Autodesk Inventor part; units mm, degrees
ref_plane "Work Plane1" through (0, 0, 5) normal (0, 0, 1) x (1, 0, 0)
ref_plane "YZ Plane" through (0, 0, 0) normal (1, 0, 0) x (0, 1, 0)
ref_plane "XZ Plane" through (0, 0, 0) normal (0, 1, 0) x (-1, 0, 0)
sketch "Sketch1" plane through (0, 0, 0) normal (0, 0, 1) x (1, 0, 0)
  line L0 (14.6962, 12.74) -> (14.6962, 0) construction
  line L1 (10.61, 12.2) -> (1.53, 12.2)
  arc A0 (1.53, 12.2) -> (0, 10.67) centre (1.53, 10.67) ccw
  line L2 (0, 10.67) -> (0, 1.53)
  arc A1 (0, 1.53) -> (1.53, 0) centre (1.53, 1.53) ccw
  line L3 (1.53, 0) -> (10.61, 0)
  arc A2 (10.61, 0) -> (12.14, 1.53) centre (10.61, 1.53) ccw
  arc A3 (12.14, 10.67) -> (10.61, 12.2) centre (10.61, 10.67) ccw
  line L4 (12.14, 10.67) -> (12.14, 1.53)
  point P0 (0, 0)
  point P1 (0, 0)
  dimension "d10" = 12.74
ref_plane "Work Plane1" through (0, 0, 5) normal (0, 0, 1) x (1, 0, 0)
sketch "Sketch2" plane through (0, 0, 5) normal (0, 0, 1) x (1, 0, 0)
  line L0 (10.88, 12.74) -> (1.8, 12.74)
  line L1 (10.88, 12.74) -> (1.8, 12.74)
  arc A0 (1.8, 12.74) -> (0, 10.94) centre (1.8, 10.94) ccw
  line L2 (0, 10.94) -> (0, 1.8)
  arc A1 (0, 1.8) -> (1.8, 0) centre (1.8, 1.8) ccw
  line L3 (1.8, 0) -> (10.88, 0)
  arc A2 (10.88, 0) -> (12.68, 1.8) centre (10.88, 1.8) ccw
  line L4 (12.68, 1.8) -> (12.68, 10.94)
  arc A3 (12.68, 10.94) -> (10.88, 12.74) centre (10.88, 10.94) ccw
  circle A4 centre (6.34, 6.37) radius 2.8
  line L5 (5.665, 8.395) -> (7.015, 8.395)
  line L6 (7.015, 4.345) -> (5.665, 4.345)
  line L7 (5.665, 4.345) -> (7.015, 8.395) construction
  line L8 (5.665, 8.395) -> (7.015, 4.345) construction
  line L9 (8.365, 5.695) -> (8.365, 7.045)
  line L10 (4.315, 7.045) -> (4.315, 5.695)
  line L11 (4.315, 5.695) -> (8.365, 7.045) construction
  line L12 (8.365, 5.695) -> (4.315, 7.045) construction
  line L13 (4.315, 5.695) -> (5.665, 5.695)
  line L14 (7.015, 5.695) -> (8.365, 5.695)
  line L15 (5.665, 4.345) -> (5.665, 5.695)
  line L16 (5.665, 7.045) -> (5.665, 8.395)
  line L17 (8.365, 7.045) -> (7.015, 7.045)
  line L18 (5.665, 7.045) -> (4.315, 7.045)
  line L19 (7.015, 8.395) -> (7.015, 7.045)
  line L20 (7.015, 5.695) -> (7.015, 4.345)
  point P0 (0, 0)
  dimension "d3" = 5.6
  dimension "d4" = 4.05
  dimension "d5" = 1.35
  dimension "d6" = 4.05
  dimension "d7" = 1.35
extrude "Extrusion3" add sketch "Sketch1" along normal blind 5
sketch "Sketch3" plane through (0, 0, 5) normal (0, 0, 1) x (1, 0, 0)
  line L0 (10.61, 12.47) -> (1.53, 12.47)
  line L1 (10.61, 12.47) -> (1.53, 12.47)
  arc A0 (1.53, 12.47) -> (-0.27, 10.67) centre (1.53, 10.67) ccw
  line L2 (-0.27, 10.67) -> (-0.27, 1.53)
  arc A1 (-0.27, 1.53) -> (1.53, -0.27) centre (1.53, 1.53) ccw
  line L3 (1.53, -0.27) -> (10.61, -0.27)
  arc A2 (10.61, -0.27) -> (12.41, 1.53) centre (10.61, 1.53) ccw
  line L4 (12.41, 1.53) -> (12.41, 10.67)
  arc A3 (12.41, 10.67) -> (10.61, 12.47) centre (10.61, 10.67) ccw
  circle A4 centre (6.07, 6.1) radius 2.8
  line L5 (5.395, 8.125) -> (6.745, 8.125)
  line L6 (6.745, 4.075) -> (5.395, 4.075)
  line L7 (5.395, 4.075) -> (6.745, 8.125) construction
  line L8 (5.395, 8.125) -> (6.745, 4.075) construction
  line L9 (8.095, 5.425) -> (8.095, 6.775)
  line L10 (4.045, 6.775) -> (4.045, 5.425)
  line L11 (4.045, 5.425) -> (8.095, 6.775) construction
  line L12 (8.095, 5.425) -> (4.045, 6.775) construction
  line L13 (4.045, 5.425) -> (5.395, 5.425)
  line L14 (6.745, 5.425) -> (8.095, 5.425)
  line L15 (5.395, 4.075) -> (5.395, 5.425)
  line L16 (5.395, 6.775) -> (5.395, 8.125)
  line L17 (8.095, 6.775) -> (6.745, 6.775)
  line L18 (5.395, 6.775) -> (4.045, 6.775)
  line L19 (6.745, 8.125) -> (6.745, 6.775)
  line L20 (6.745, 5.425) -> (6.745, 4.075)
  line L21 (10.61, 12.2) -> (1.53, 12.2)
  line L22 (0, 10.67) -> (0, 1.53)
  point P0 (0, 0)
  point P1 (-0.27, -0.27)
  point P2 (6.07, 12.2)
  point P3 (0, 6.1)
  point P4 (6.07, 6.1)
  dimension "d14" = 5.6
  dimension "d15" = 4.05
  dimension "d16" = 1.35
  dimension "d17" = 4.05
  dimension "d18" = 1.35
extrude "Extrusion4" add sketch "Sketch3" along normal blind 4.8 contours A4
sketch "Sketch4" plane through (0, 0, 0) normal (0, 0, -1) x (-1, 0, 0)
  line L0 (-13.9436, 0) -> (-13.9436, 2.266)
  line L1 (-15.5559, 0) -> (-15.5559, 6.84)
  line L2 (-1.53, 0) -> (-10.61, 0)
  line L3 (-11.5311, 9.89) -> (-0.6089, 9.89) construction
  line L4 (-0.6089, 9.89) -> (-0.6089, 6.84) construction
  line L5 (-0.6089, 6.84) -> (-11.5311, 6.84) construction
  line L6 (-11.5311, 6.84) -> (-11.5311, 9.89) construction
  line L7 (-7.4059, 5.4371) -> (-4.7341, 5.4371) construction
  line L8 (-4.7341, 5.4371) -> (-4.7341, 2.266) construction
  line L9 (-4.7341, 2.266) -> (-7.4059, 2.266) construction
  line L10 (-7.4059, 2.266) -> (-7.4059, 5.4371) construction
  line L11 (-10.6289, 6.84) -> (-10.6289, 9.3092)
  line L12 (-10.6289, 9.3092) -> (-11.5311, 9.3092)
  line L13 (-11.5311, 9.3092) -> (-11.5311, 9.89)
  line L14 (-11.5311, 9.89) -> (-8.9606, 9.89)
  line L15 (-8.9606, 9.89) -> (-8.9606, 9.3092)
  line L16 (-8.9606, 9.3092) -> (-9.8627, 9.3092)
  line L17 (-9.8627, 9.3092) -> (-9.8627, 6.84)
  line L18 (-9.8627, 6.84) -> (-10.6289, 6.84)
  line L19 (-7.1291, 6.84) -> (-8.7703, 6.84)
  line L20 (-8.7703, 6.84) -> (-8.7703, 7.3714)
  line L21 (-8.7703, 7.3714) -> (-8.3328, 7.3714)
  line L22 (-8.3328, 7.3714) -> (-8.3328, 9.3586)
  line L23 (-8.3328, 9.3586) -> (-8.7703, 9.3586)
  line L24 (-8.7703, 9.3586) -> (-8.7703, 9.89)
  line L25 (-8.7703, 9.89) -> (-7.1291, 9.89)
  line L26 (-7.1291, 9.89) -> (-7.1291, 9.3586)
  line L27 (-7.1291, 9.3586) -> (-7.5666, 9.3586)
  line L28 (-7.5666, 9.3586) -> (-7.5666, 7.3714)
  line L29 (-7.5666, 7.3714) -> (-7.1291, 7.3714)
  line L30 (-7.1291, 7.3714) -> (-7.1291, 6.84)
  line L31 (-3.5057, 6.84) -> (-4.2669, 6.84)
  line L32 (-4.2669, 6.84) -> (-4.2669, 8.8618)
  line L33 (-4.2669, 8.8618) -> (-4.8206, 7.5568)
  line L34 (-4.8206, 7.5568) -> (-5.3446, 7.5568)
  line L35 (-5.3446, 7.5568) -> (-5.8982, 8.8618)
  line L36 (-5.8982, 8.8618) -> (-5.8982, 6.84)
  line L37 (-5.8982, 6.84) -> (-6.6199, 6.84)
  line L38 (-6.6199, 6.84) -> (-6.6199, 9.89)
  line L39 (-6.6199, 9.89) -> (-5.7376, 9.89)
  line L40 (-5.7376, 9.89) -> (-5.0603, 8.3848)
  line L41 (-5.0603, 8.3848) -> (-4.3881, 9.89)
  line L42 (-4.3881, 9.89) -> (-3.5057, 9.89)
  line L43 (-3.5057, 9.89) -> (-3.5057, 6.84)
  line L44 (-2.8729, 6.84) -> (-2.8729, 9.89)
  line L45 (-2.8729, 9.89) -> (-0.8116, 9.89)
  line L46 (-0.8116, 9.89) -> (-0.8116, 9.3092)
  line L47 (-0.8116, 9.3092) -> (-2.1117, 9.3092)
  line L48 (-2.1117, 9.3092) -> (-2.1117, 8.7728)
  line L49 (-2.1117, 8.7728) -> (-0.9129, 8.7728)
  line L50 (-0.9129, 8.7728) -> (-0.9129, 8.192)
  line L51 (-0.9129, 8.192) -> (-2.1117, 8.192)
  line L52 (-2.1117, 8.192) -> (-2.1117, 7.4208)
  line L53 (-2.1117, 7.4208) -> (-0.8116, 7.4208)
  line L54 (-0.8116, 7.4208) -> (-0.8116, 6.84)
  line L55 (-0.8116, 6.84) -> (-2.8729, 6.84)
  spline S0 degree 2 poles (-4.8725, 3.3684) (-4.8725, 2.8864) (-5.483, 2.266) (-6.0169, 2.266) knots 0 0 0 1 2 2 2
  spline S1 degree 2 poles (-6.0169, 2.266) (-6.2838, 2.266) (-6.7015, 2.4192) (-6.8473, 2.57) knots 0 0 0 1 2 2 2
  spline S2 degree 2 poles (-6.8473, 2.57) (-7.0203, 2.7455) (-7.2057, 3.3016) (-7.2057, 3.6897) knots 0 0 0 1 2 2 2
  spline S3 degree 2 poles (-7.2057, 3.6897) (-7.2057, 4.0901) (-7.0327, 4.7129) (-6.8374, 4.9527) knots 0 0 0 1 2 2 2
  spline S4 degree 2 poles (-6.8374, 4.9527) (-6.6521, 5.1801) (-6.049, 5.4371) (-5.6362, 5.4371) knots 0 0 0 1 2 2 2
  spline S5 degree 2 poles (-5.6362, 5.4371) (-5.4855, 5.4371) (-5.1839, 5.3976) (-5.1295, 5.3852) knots 0 0 0 1 2 2 2
  line L56 (-5.1295, 5.3852) -> (-5.1295, 4.7871)
  line L57 (-5.1295, 4.7871) -> (-5.1839, 4.7871)
  spline S6 degree 2 poles (-5.1839, 4.7871) (-5.2383, 4.8143) (-5.4855, 4.881) (-5.6436, 4.881) knots 0 0 0 1 2 2 2
  spline S7 degree 2 poles (-5.6436, 4.881) (-6.002, 4.881) (-6.3925, 4.5028) (-6.4395, 4.1519) knots 0 0 0 1 2 2 2
  spline S8 degree 2 poles (-6.4395, 4.1519) (-6.2887, 4.2483) (-5.9798, 4.3619) (-5.7845, 4.3619) knots 0 0 0 1 2 2 2
  spline S9 degree 2 poles (-5.7845, 4.3619) (-5.6189, 4.3619) (-5.3297, 4.273) (-5.2185, 4.1889) knots 0 0 0 1 2 2 2
  spline S10 degree 2 poles (-5.2185, 4.1889) (-5.0603, 4.0678) (-4.8725, 3.6748) (-4.8725, 3.3684) knots 0 0 0 1 2 2 2
  spline S11 degree 2 poles (-5.7648, 2.9086) (-5.7054, 2.9828) (-5.6412, 3.1558) (-5.6412, 3.3313) knots 0 0 0 1 2 2 2
  spline S12 degree 2 poles (-5.6412, 3.3313) (-5.6412, 3.4796) (-5.7153, 3.6724) (-5.7821, 3.7292) knots 0 0 0 1 2 2 2
  spline S13 degree 2 poles (-5.7821, 3.7292) (-5.8513, 3.7885) (-6.0218, 3.8305) (-6.1182, 3.8305) knots 0 0 0 1 2 2 2
  spline S14 degree 2 poles (-6.1182, 3.8305) (-6.1998, 3.8305) (-6.3678, 3.7885) (-6.442, 3.7589) knots 0 0 0 1 2 2 2
  spline S15 degree 2 poles (-6.442, 3.7589) (-6.442, 3.7391) (-6.4469, 3.6452) (-6.4469, 3.5735) knots 0 0 0 1 2 2 2
  spline S16 degree 2 poles (-6.4469, 3.5735) (-6.4469, 3.309) (-6.3555, 2.9902) (-6.2838, 2.9086) knots 0 0 0 1 2 2 2
  spline S17 degree 2 poles (-6.2838, 2.9086) (-6.2319, 2.8419) (-6.0935, 2.785) (-6.0193, 2.785) knots 0 0 0 1 2 2 2
  spline S18 degree 2 poles (-6.0193, 2.785) (-5.9575, 2.785) (-5.8142, 2.8468) (-5.7648, 2.9086) knots 0 0 0 1 2 2 2
  point P0 (0, 0)
  point P1 (-6.07, 0)
  point P2 (-6.07, 2.266)
  point P3 (-6.07, 6.84)
  point P4 (-6.07, 6.84)
  point P5 (-6.07, 2.266)
  dimension "d21" = 2.266
  dimension "d22" = 6.84
extrude "Extrusion5" add sketch "Sketch4" along normal blind 0.9
properties part number "IPC TIME 6 key"
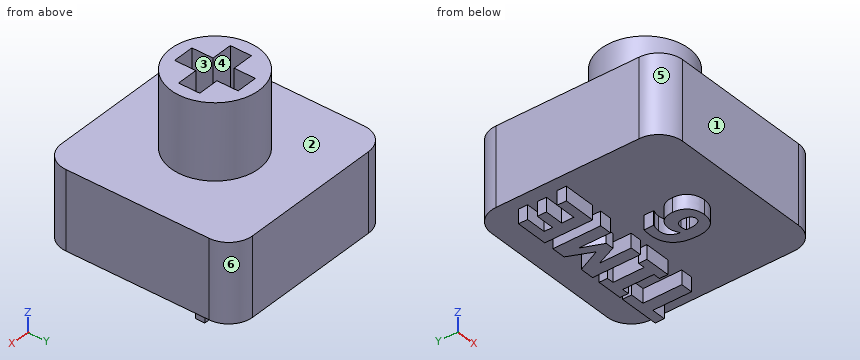
Check sheet for the modelled part. Datum: model origin and axes. Units: mm. Face numbers are marked on the shaded views. A direction names the side the tool comes from. Round coordinates to 2 decimals unless told otherwise and drop trailing zeros. Order: outer loops, then holes, each group sorted by start corner. A loop starts at its lowest first (then second) coordinate and runs counter-clockwise, first axis right, second up. Notation, with made-up numbers: (66, 8.25) -> (119, 8.25) arc R19 ccw to (119, 43.25) -> close; hole circle Ø9 at (24.5, 53). An arc over 180 degrees is marked (long way). One line per item, written item: value. Start each with the question number.
Q1. Cross-section at B-B (y = 6.1). Record the boundary of the cut face in (x, z) (3 decimals), and give its area (3 significant figures).
Q2. Thickness scan on line 1 (Z direction, x = 9.25, y = 1); line 2 (Z direction, x = 7.25, y = 4); line 3 (X direction, y = 8.5, z = 8). Record the ranges inside material, lowest first.
Q3. Set-up check for the marked faces 1 and 2: record each of +Z, -Z, +X, -X, +Y, -Y from which the full face is reachable in a straight line by a thin tool's end or side.
Q4. Cross-section at A-A (z = 5.5). Record the boundary of the cut face in (x, y) (3 decimals), and give its area (3 significant figures).
Q5. Gauge pin test, flat ends, axial feed: pin 1 Ø0.7 at (x, z) = (4.5, 8) entering from +Y; pin 2 Ø0.7 at (y, z) = (8, -0.5) entering from +X; pin 3 Ø0.7 at (x, z) = (4.5, 7) entering from -Y. Record the tip position at first contact, or that the pin passes through.
Q6. Mould release check, pull along Y, two halves, no side actions. Record for the marked faces 3, 4, 5 and 6: pulls with the +Y half, pulls with the -Y half, needs draft (parallel to the pull), parting line crosses it, or undercut.
Completed:
1. outline: (0, 0) -> (12.14, 0) -> (12.14, 5) -> (8.87, 5) -> (8.87, 9.8) -> (8.095, 9.8) -> (8.095, 5) -> (4.045, 5) -> (4.045, 9.8) -> (3.27, 9.8) -> (3.27, 5) -> (0, 5) -> close
1. area: 68.1 mm²
2. line 1: z = 0 to 5
2. line 2: z = 0 to 9.8
2. line 3: x = 4.63 to 7.51
3. face 1: +Z, -Z, +X, -X, -Y
3. face 2: +Z
4. outline: circle Ø5.6 at (6.07, 6.1); hole (4.045, 5.425) -> (5.395, 5.425) -> (5.395, 4.075) -> (6.745, 4.075) -> (6.745, 5.425) -> (8.095, 5.425) -> (8.095, 6.775) -> (6.745, 6.775) -> (6.745, 8.125) -> (5.395, 8.125) -> (5.395, 6.775) -> (4.045, 6.775) -> close
4. area: 15.5 mm²
5. pin 1: stops at y = 8.62
5. pin 2: stops at x = 10.63
5. pin 3: stops at y = 3.58
6. face 3: undercut
6. face 4: undercut
6. face 5: pulls with the -Y half
6. face 6: pulls with the +Y half
